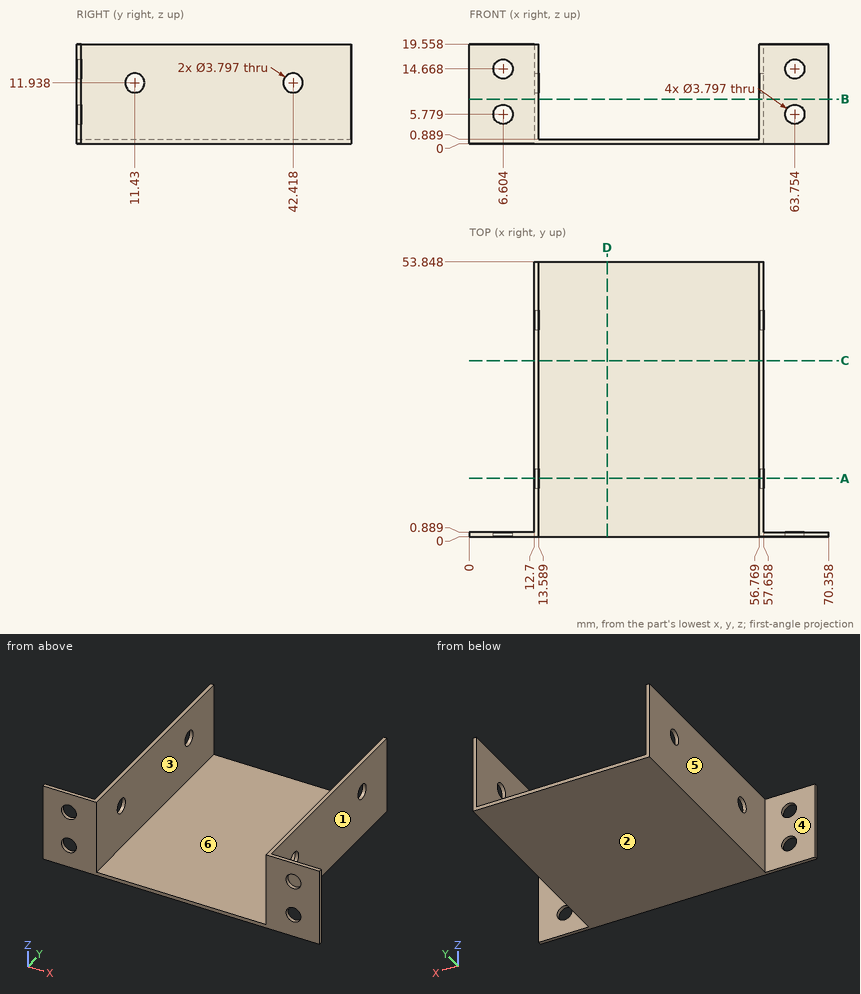
Verification items for this drawing (mm, ordinates from the low corner). A direction names the side the tool comes from. Round coordinates to 2 decimals unless told otherwise and drop trailing zeros. Write each loop counter-clockwise with the first axis right and the second up, starting at its lowest first coordinate (ties: lowest second). Pieces come first, ordered by that corner, then holes. Notation, with made-up numbers: (40.5, 42) - (81.5, 42) arc R30 ccw to (81.5, 71) - close; hole circle Ø11 at (40.25, -13). An arc over 180 degrees is marked (long way). One line per item, written item: value.
1. Cross-section at B-B on z = 8.75. Record the boundary of the cut face in (x, y).
The answers:
outline: (0, 0) - (13.59, 0) - (13.59, 53.85) - (12.7, 53.85) - (12.7, 0.89) - (0, 0.89) - close; (56.77, 0) - (70.36, 0) - (70.36, 0.89) - (57.66, 0.89) - (57.66, 53.85) - (56.77, 53.85) - close
2. Cross-section at D-D on x = 27. Record the boundary of the cut face in (y, z).
The answers:
outline: (0, 0) - (53.85, 0) - (53.85, 0.89) - (0, 0.89) - close
3. Scan lines: L1, parallel to X at y = 25.5, z = 13.75; L2, parallel to Z at x = 40.5, y = 35. Record each from-to range of solid material in increasing order.
The answers:
L1: x = 12.7 to 13.59, 56.77 to 57.66
L2: z = 0 to 0.89
4. Cross-section at C-C on y = 34.5. Record the boundary of the cut face in (x, z).
The answers:
outline: (12.7, 0) - (57.66, 0) - (57.66, 19.56) - (56.77, 19.56) - (56.77, 0.89) - (13.59, 0.89) - (13.59, 19.56) - (12.7, 19.56) - close
5. Mould release check, pull along X, two halves, no side actions. Record for the marked faces 4, 5 and 6: released by +X, released by -X, zero draft, split by the parting line, or undercut.
The answers:
face 4: zero draft
face 5: released by -X
face 6: undercut
6. Cross-section at A-A on y = 11.43. Record the boundary of the cut face in (x, z).
The answers:
outline: (12.7, 0) - (57.66, 0) - (57.66, 10.04) - (56.77, 10.04) - (56.77, 0.89) - (13.59, 0.89) - (13.59, 10.04) - (12.7, 10.04) - close; (12.7, 13.84) - (13.59, 13.84) - (13.59, 19.56) - (12.7, 19.56) - close; (56.77, 13.84) - (57.66, 13.84) - (57.66, 19.56) - (56.77, 19.56) - close
7. Set-up check for the marked faces 1, 2 and 3: record each of +Z, -Z, +X, -X, +Y, -Y from which the full face is reachable in a straight line by a thin tool's end or side.
The answers:
face 1: +Z, -Z, +X, +Y
face 2: -Z, +X, -X, +Y, -Y
face 3: +Z, +Y, -Y
8. Depth check by flat-ended pin: pin 1 Ø3.5 at (y, z) = (11.43, 11.938) entering from +X; pin 2 Ø1.5 at (y, z) = (7.5, 13.5) entering from +X; pin 3 Ø1 at (x, y) = (50.5, 13.5) entering from -Z; pin 4 Ø6.5 at (x, z) = (64, 14) entering from +Y. Enter the tip coordinate at first touch or a pass-through.
The answers:
pin 1: passes through
pin 2: stops at x = 57.66
pin 3: stops at z = 0
pin 4: stops at y = 0.89
